from build123d import *

# Parameters (mm, degrees)
ESBO_O1_R                = 12.2
RESSALTO_EXTRUS_O1_DEPTH = 30.8
FILETE1_R                = 1
ESBO_O2_R                = 2
RESSALTO_EXTRUS_O2_DEPTH = 10
ESBO_O4_W                = 0.958903526
ESBO_O4_H                = 3.564219336
ESBO_O4_W_2              = 0.894406544
RESSALTO_EXTRUS_O3_DEPTH = 5
FILETE2_R                = 1
ESBO_O5_R                = 0.782109668
CORTE_EXTRUS_O2_DEPTH    = 22.982815538
ESBO_O6_R                = 5
RESSALTO_EXTRUS_O5_DEPTH = 10
INCLINA_O3_ANGLE         = 30


with BuildPart() as part:
    # Esboço1 → Ressalto-extrusão1 (new body)
    with BuildSketch(Plane.XY):
        Circle(ESBO_O1_R)
    extrude(amount=RESSALTO_EXTRUS_O1_DEPTH)

    # Filete1
    filete1_edges = [part.edges().sort_by_distance(p)[0] for p in [
        (-12.2, 0, 0),
        (-12.2, 0, 30.8),
    ]]
    fillet(filete1_edges, radius=FILETE1_R)

    # Esboço2 → Ressalto-extrusão2 (add)
    with BuildSketch(Plane.XY.offset(30.8)):
        Circle(ESBO_O2_R)
    extrude(amount=RESSALTO_EXTRUS_O2_DEPTH)

    # Esboço4 → Ressalto-extrusão3 (add)
    with BuildSketch(Plane(origin=(0, 0, 0), x_dir=(-1, 0, 0), z_dir=(0, 0, -1))):
        with Locations((-9.303363775, 0.548104497)):
            Rectangle(ESBO_O4_W, ESBO_O4_H)
        with Locations((8.369776419, 0.548104497)):
            Rectangle(ESBO_O4_W_2, ESBO_O4_H)
    extrude(amount=RESSALTO_EXTRUS_O3_DEPTH)

    # Filete2
    filete2_edges = [part.edges().sort_by_distance(p)[0] for p in [
        (9.303363775, -1.234005171, -5),
        (9.303363775, 2.330214165, -5),
        (-8.369776419, 2.330214165, -5),
        (-8.369776419, -1.234005171, -5),
    ]]
    fillet(filete2_edges, radius=FILETE2_R)

    # Esboço5 → Corte-extrusão2 (cut, through all)
    with BuildSketch(Plane(origin=(9.782815538, 0, 0), x_dir=(0, 0, -1), z_dir=(1, 0, 0))):
        with Locations((3.47716986, 0.548104497)):
            Circle(ESBO_O5_R)
    extrude(amount=-CORTE_EXTRUS_O2_DEPTH, mode=Mode.SUBTRACT)

    # Esboço6 → Ressalto-extrusão5 (add)
    with BuildSketch(Plane.XY.offset(40.8)):
        Circle(ESBO_O6_R)
    extrude(amount=RESSALTO_EXTRUS_O5_DEPTH)

    # Inclinação3
    inclina_o3_faces = [part.faces().sort_by_distance(p)[0] for p in [
        (-5, 0, 45.8),
    ]]
    draft(inclina_o3_faces, Plane.XY.offset(50.8), INCLINA_O3_ANGLE)


solid = part.part
Source: CAD feature listing. Evaluate the final solid. Frame: model axes, mm. A direction names the side the tool comes from. Give positions to 0.01 mm unless a question says otherwise; leave off trailing zeros. Write each loop counter-clockwise with the first axis right and the second up, starting at its lowest first coordinate (ties: lowest second). Pieces come first, ordered by that corner, then holes. Notation, with made-up numbers: M -22,20.5 L 23,20.5 A32 cw 23,58.5 Z; hole C 55,-15 d7. An arc over 180 degrees is marked long. Return JSON: item names as keys, results as strings. Group by question number.
1) Cut plane B-B, the plane z = 3.5. Output: boundary loops of the cut face in (x, y), then the cut area to 3 significant figures.
2) Set-up query: faces 1 (the face through (-8.817, 1, -2)), 2 (the face through (9.783, 1, -2)), 3 (the face through (8.824, 1, -2)), 4 (the face through (0, -2, 36)). Return all of +Z, -Z, +X, -X, +Y, -Y with unobstructed straight access to the full face (end or side cutting, diameter ignored); none if empty.
3) Draft query along X for faces 5 (the face through (5.73, 1.8, 49.06)), 6 (the face through (-7.923, 1, -2)), 7 (the face through (2.2, 0.2, 40.8)). Return one class per face: released by +X, released by -X, zero draft, split by the parting line, or undercut.
4) Ray query, L1, parallel to Z at x = 1, y = 3.5; L2, parallel to Z at x = 10, y = 4.25; L3, parallel to Z at x = -8.75, y = -4.25. Return the intervals inside material, ascending.
5) First-contact query: pin 1 Ø1.5 at (x, z) = (5, 2) entering from +Y; pin 2 Ø1.3 at (y, z) = (0.55, -3.48) entering from +X; pin 3 Ø2 at (x, y) = (-8, -1.5) entering from +Z; pin 4 Ø1 at (x, z) = (-8.5, -2.5) entering from -Y. Flat tips, straight axial feed; report the tip coordinate or a pass-through.
6) Cut plane C-C, the plane z = 45.5. Output: boundary loops of the cut face in (x, y), then the cut area to 3 significant figures.
7) Cut plane A-A, the plane x = 0. Output: boundary loops of the cut face in (y, z), then the cut area to 3 significant figures.
Data:
{
 "1": {"outline": "C 0,0 d24.4", "area": "468 mm²"},
 "2": {"face 1": "-Z, -X, +Y, -Y", "face 2": "-Z, +X, +Y, -Y", "face 3": "-Z, +Y, -Y", "face 4": "none"},
 "3": {"face 5": "split by the parting line", "face 6": "undercut", "face 7": "zero draft"},
 "4": {"L1": "z = 0 to 30.8, 40.8 to 50.8", "L2": "z = 0 to 30.8", "L3": "z = 0 to 30.8, 40.8 to 42.61"},
 "5": {"pin 1": "stops at y = 11.44", "pin 2": "passes through", "pin 3": "stops at z = 47.09", "pin 4": "stops at y = -1.23"},
 "6": {"outline": "C 0,0 d16.12", "area": "204 mm²"},
 "7": {"outline": "M -12.2,1 A1 ccw -11.2,0 L 11.2,0 A1 ccw 12.2,1 L 12.2,29.8 A1 ccw 11.2,30.8 L 2,30.8 L 2,40.8 L 10.77,40.8 L 5,50.8 L -5,50.8 L -10.77,40.8 L -2,40.8 L -2,30.8 L -11.2,30.8 A1 ccw -12.2,29.8 Z", "area": "948 mm²"}
}
